```python
from build123d import *

# Parameters (mm, degrees)
SKETCH1_W         = 44.45
SKETCH1_H         = 30.9626
EXTRUDE1_DEPTH    = 17.4752
SKETCH2_W         = 41.3004
SKETCH2_H         = 29.3878
EXTRUDE2_DEPTH    = 17.4752
SKETCH3_OUTSIDE_W = 30.859
SKETCH3_OUTSIDE_H = 44.347
EXTRUDE3_DEPTH    = 45.45
SKETCH4_R         = 4.0005
SKETCH4_R_2       = 1.1938
EXTRUDE4_DEPTH    = 45.45
SKETCH5_R         = 4.0005
SKETCH5_R_2       = 1.1938
EXTRUDE5_DEPTH    = 17.4752
FILLET1_R         = 1.5748
FILLET2_R         = 0.254


with BuildPart() as part:
    # Sketch1 → Extrude1 (new body)
    with BuildSketch(Plane(origin=(0, 0, 0), x_dir=(0, 0, -1), z_dir=(1, 0, 0))):
        with Locations((22.225, 15.4813)):
            Rectangle(SKETCH1_W, SKETCH1_H)
    extrude(amount=EXTRUDE1_DEPTH)

    # Sketch2 → Extrude2 (cut)
    with BuildSketch(Plane(origin=(17.4752, 0, 0), x_dir=(0, 0, -1), z_dir=(1, 0, 0))):
        with Locations((22.225, 16.2687)):
            Rectangle(SKETCH2_W, SKETCH2_H)
    extrude(amount=-EXTRUDE2_DEPTH, mode=Mode.SUBTRACT)

    # Sketch3 outside → Extrude3 (cut, through all)
    with BuildSketch(Plane.XY):
        with Locations((8.7375, 15.4815)):
            Rectangle(SKETCH3_OUTSIDE_W, SKETCH3_OUTSIDE_H)
        with BuildLine():
            Line((0, 22.225), (0, 0))
            Line((0, 0), (17.4752, 0))
            Line((17.4752, 0), (17.4752, 22.225))
            ThreePointArc((17.4752, 22.225), (8.7376, 30.9626), (0, 22.225))
        make_face(mode=Mode.SUBTRACT)
    extrude(amount=-EXTRUDE3_DEPTH, mode=Mode.SUBTRACT)

    # Sketch4 → Extrude4 (cut, through all)
    with BuildSketch(Plane.XY):
        with Locations((8.7376, 22.225)):
            Circle(SKETCH4_R)
        with Locations((2.4765, 22.225)):
            Circle(SKETCH4_R_2)
        with Locations((14.9987, 22.225)):
            Circle(SKETCH4_R_2)
        with Locations((8.7376, 15.9639)):
            Circle(SKETCH4_R_2)
        with Locations((8.7376, 28.4861)):
            Circle(SKETCH4_R_2)
    extrude(amount=-EXTRUDE4_DEPTH, mode=Mode.SUBTRACT)

    # Sketch5 → Extrude5 (cut)
    with BuildSketch(Plane(origin=(0, 1.5748, 0), x_dir=(1, 0, 0), z_dir=(0, 1, 0))):
        with Locations(Location((8.7376, 22.225, 0), (0, 0, 270))):  # turned: the seam where the file's is
            Circle(SKETCH5_R)
        with Locations(Location((2.4765, 22.225, 0), (0, 0, 270))):  # turned: the seam where the file's is
            Circle(SKETCH5_R_2)
        with Locations(Location((14.9987, 22.225, 0), (0, 0, 270))):  # turned: the seam where the file's is
            Circle(SKETCH5_R_2)
        with BuildLine():
            Line((9.9314, 30.5562), (9.9314, 28.4861))
            ThreePointArc((9.9314, 28.4861), (8.7376, 27.2923), (7.5438, 28.4861))
            Line((7.5438, 28.4861), (7.5438, 30.5562))
            ThreePointArc((7.5438, 30.5562), (8.7376, 31.75), (9.9314, 30.5562))
        make_face()
        with BuildLine():
            Line((7.5438, 15.9639), (7.5438, 13.8684))
            ThreePointArc((7.5438, 13.8684), (8.7376, 12.6746), (9.9314, 13.8684))
            Line((9.9314, 13.8684), (9.9314, 15.9639))
            ThreePointArc((9.9314, 15.9639), (8.7376, 17.1577), (7.5438, 15.9639))
        make_face()
    extrude(amount=-EXTRUDE5_DEPTH, mode=Mode.SUBTRACT)

    # Fillet1
    fillet1_edges = [part.edges().sort_by_distance(p)[0] for p in [
        (8.7376, 0, -44.45),
        (8.7376, 0, 0),
    ]]
    fillet(fillet1_edges, radius=FILLET1_R)

    # Fillet2
    fillet2_edges = [part.edges().sort_by_distance(p)[0] for p in [
        (8.7376, 1.5748, -42.8752),
        (8.7376, 1.5748, -1.5748),
    ]]
    fillet(fillet2_edges, radius=FILLET2_R)


solid = part.part
```
Work out the finished part from the listing and answer in its coordinate system (mm). A direction names the side the tool comes from. Round coordinates to 2 decimals unless told otherwise and drop trailing zeros. Order: outer loops, then holes, each group sorted by start corner. A loop starts at its lowest first (then second) coordinate and runs counter-clockwise, first axis right, second up.
Q1. Given pin 1 Ø4 at (x, z) = (6, -15.5) entering from +Y, flat-ended and moving along its own axis, determine where the tip first touches the part or whether it passes through.
Solution:
pin 1: stops at y = 1.57
Q2. A cutting plane is placed at C-C, the plane x = 6.5. Determine the outline of the cut face in (y, z), then the cut area to 3 significant figures.
Solution:
outline: (0, -42.88) arc R1.57 ccw to (1.57, -44.45) - (18.91, -44.45) - (18.91, -42.88) - (1.83, -42.88) arc R0.25 cw to (1.57, -42.62) - (1.57, -25.54) - (0, -25.54) - close; (0, -18.91) - (1.57, -18.91) - (1.57, -1.83) arc R0.25 cw to (1.83, -1.57) - (18.91, -1.57) - (18.91, 0) - (1.57, 0) arc R1.57 ccw to (0, -1.57) - close; (25.54, -44.45) - (30.67, -44.45) - (30.67, -42.88) - (25.54, -42.88) - close; (25.54, -1.57) - (30.67, -1.57) - (30.67, 0) - (25.54, 0) - close
area: 129 mm2
Q3. Find the intervals of material crossed by line 1 along Z through (x, y) = (5.25, 8); line 2 along Y through (x, z) = (15, -9), in increasing order.
Solution:
line 1: z = -44.45 to -42.88, -1.57 to 0
line 2: y = 0 to 1.57
Q4. A tool of negligible diameter and unlimited length cuts with its end or side. For faces 1 (the cylindrical face through (8.764, 0.798, -17.157)), 2 (the cylindrical face through (3.027, 21.166, -0.776)), 3 (the flat face through (9, 13, -42.875)), from which of +Z, -Z, +X, -X, +Y, -Y can it reach the whole face along a straight path? Write none if from no direction.
Solution:
face 1: +Y, -Y
face 2: +Z, -Z
face 3: +X, -X, +Y
Q5. A cutting plane is placed at A-A, the plane z = -14.5. Determine the outline of the cut face in (x, y).
Solution:
outline: (0, 0) - (7.54, 0) - (7.54, 1.57) - (0, 1.57) - close; (9.93, 0) - (17.48, 0) - (17.48, 1.57) - (9.93, 1.57) - close
Q6. The mould has two halves that part along Z. Classify faces 4 (the flat face through (7.544, 1, -30)), 5 (the cylindrical face through (14.05, 21.5, -0.78)), 6 (the flat face through (9, 13, 0)): pulls with the +Z half, pulls with the -Z half, needs draft (parallel to the pull), parting line crosses it, or undercut.
Solution:
face 4: undercut
face 5: needs draft
face 6: pulls with the +Z half
Q7. A cutting plane is placed at D-D, the plane y = 10.5. Determine the outline of the cut face in (x, z).
Solution:
outline: (0, -44.45) - (17.48, -44.45) - (17.48, -42.88) - (0, -42.88) - close; (0, -1.57) - (17.48, -1.57) - (17.48, 0) - (0, 0) - close
Q8. A cutting plane is placed at B-B, the plane y = 29. Determine the outline of the cut face in (x, z).
Solution:
outline: (3.22, -44.45) - (7.66, -44.45) - (7.66, -42.88) - (3.22, -42.88) - close; (3.22, -1.57) - (7.66, -1.57) - (7.66, 0) - (3.22, 0) - close; (9.82, -44.45) - (14.26, -44.45) - (14.26, -42.88) - (9.82, -42.88) - close; (9.82, -1.57) - (14.26, -1.57) - (14.26, 0) - (9.82, 0) - close
